Verification items for the finished model (mm, model axes). A direction names the side the tool comes from. Give positions to 0.01 mm unless a question says otherwise; leave off trailing zeros. Loops run counter-clockwise (first coordinate to the right, second up) from the corner with the lowest first, then second, coordinate; pieces in that order, holes last. Notation, with made-up numbers: M 53.25,33 L 92.25,33 A32 cw 92.25,69 Z; hole C 29.5,89.5 d5. An arc over 180 degrees is marked long. Answer in a Markdown table with one row per item.
```python
from build123d import *

# Parameters (mm, degrees)
F0_R     = 76.2
F1_DEPTH = 25.4
F2_R     = 50.8
F3_DEPTH = 25.4
F4_W     = 9.9899098277
F4_H     = 8.6538987234
F5_DEPTH = 25.4


# Not quite as in the source:
# - a feature names something its author has since deleted; it is built from what else it names


with BuildPart() as f1:
    # F0 (on Right) → F1 (new body)
    with BuildSketch(Plane.YZ):
        Circle(F0_R)
    extrude(amount=F1_DEPTH)

    # F2 (on face) → F3 (cut)
    with BuildSketch(Plane.YZ.offset(25.4)):
        Circle(F2_R)
    extrude(amount=-F3_DEPTH, mode=Mode.SUBTRACT)

    # F4 (on face) → F5 (cut)
    with BuildSketch(Plane(origin=(0, 0, 0), x_dir=(0, -1, 0), z_dir=(-1, 0, 0))):
        with Locations((-58.8261894882, 17.9770062678)):
            Rectangle(F4_W, F4_H)
    extrude(amount=-F5_DEPTH, mode=Mode.SUBTRACT)


solid = f1.part
```
Item 1: Sectioned sample at A-A (y = 0). Record the cut outline in (x, z).
Reported:
| item | result |
|---|---|
| outline | M 0,-76.2 L 25.4,-76.2 L 25.4,-50.8 L 0,-50.8 Z; M 0,50.8 L 25.4,50.8 L 25.4,76.2 L 0,76.2 Z |
Item 2: Sectioned sample at C-C (x = 2). Record the cut outline in (y, z), and give its area (3 significant figures).
Reported:
| item | result |
|---|---|
| outline | C 0,0 d152.4; hole C 0,0 d101.6; hole M 53.83,13.65 L 63.82,13.65 L 63.82,22.3 L 53.83,22.3 Z |
| area | 10,000 mm^2 |
Item 3: Go/stop test with flat-tipped pins: pin 1 (9.5 mm diameter, centred on x = 9, z = 20, fed in from +Y); pin 2 (9.5 mm diameter, centred on x = 12, z = 18, fed in from -Y); pin 3 (8 mm diameter, centred on x = 22, y = 4.5, fed in from +Z). Record where each tip stops, or that it passes through.
Reported:
| item | result |
|---|---|
| pin 1 | stops at y = 74.66 |
| pin 2 | stops at y = -75.04 |
| pin 3 | stops at z = 76.2 |
Item 4: Release check for a two-part mould opening along Y. For faces 3 (the flat face through (13, 63.821, 18)), 4 (the flat face through (25.4, 16, -50)), 5 (the cylindrical face through (12.522, -60.47, -46.367)) record: released by +Y, released by -Y, zero draft, split by the parting line, or undercut.
Reported:
| item | result |
|---|---|
| face 3 | undercut |
| face 4 | zero draft |
| face 5 | split by the parting line |
Item 5: Tool access check on faces 1 (the flat face through (0, 16, -50)), 2 (the flat face through (13, 53.831, 18)). Record the directions out of +Z, -Z, +X, -X, +Y, -Y that give a thin tool (end or side, any length) a straight path to the whole face; none if there is none.
Reported:
| item | result |
|---|---|
| face 1 | +Z, -Z, -X, +Y, -Y |
| face 2 | +X, -X |
Item 6: Scan lines: L1, parallel to Z at x = 9.5, y = 0; L2, parallel to Y at x = 8.5, z = 6; L3, parallel to Z at x = 15, y = 59. Record each from-to range of solid material in increasing order. Write a range as [from, to].
Reported:
| item | result |
|---|---|
| L1 | z = [-76.2, -50.8], [50.8, 76.2] |
| L2 | y = [-75.96, -50.44], [50.44, 75.96] |
| L3 | z = [-48.22, 13.65], [22.3, 48.22] |
